Geometry: final body of the model. Coordinates: model frame, mm. Face numbers are marked on the shaded views. A direction names the side the tool comes from. Give positions to 0.01 mm unless a question says otherwise; leave off trailing zeros. Loops run counter-clockwise (first coordinate to the right, second up) from the corner with the lowest first, then second, coordinate; pieces in that order, holes last.
from build123d import *

# Parameters (mm, degrees)
SKETCH4_W                     = 38.1
SKETCH4_H                     = 38.1
BOSS_EXTRUDE2_DEPTH           = 15.24
BOSS_EXTRUDE2_TAPER           = 45
BOSS_EXTRUDE2_OTHER_WAY_DEPTH = 19.05
SKETCH10_W                    = 50.8
SKETCH10_H                    = 50.8
BOSS_EXTRUDE3_DEPTH           = 12.7
BOSS_EXTRUDE3_TAPER           = -45
BOSS_EXTRUDE3_OTHER_WAY_DEPTH = 2.54
BOSS_EXTRUDE3_OTHER_WAY_TAPER = 45


with BuildPart() as part:
    # Sketch4 → Boss-Extrude2 (new body)
    with BuildSketch(Plane(origin=(0, 0, 0), x_dir=(0, 0, -1), z_dir=(1, 0, 0))):
        Rectangle(SKETCH4_W, SKETCH4_H)
    extrude(amount=BOSS_EXTRUDE2_DEPTH, taper=BOSS_EXTRUDE2_TAPER)

    # Sketch4 → Boss-Extrude2 other way (add)
    with BuildSketch(Plane(origin=(0, 0, 0), x_dir=(0, 0, -1), z_dir=(1, 0, 0))):
        Rectangle(SKETCH4_W, SKETCH4_H)
    extrude(amount=-BOSS_EXTRUDE2_OTHER_WAY_DEPTH)

    # Sketch10 → Boss-Extrude3 (add)
    with BuildSketch(Plane.ZY.offset(19.05)):
        Rectangle(SKETCH10_W, SKETCH10_H)
    extrude(amount=BOSS_EXTRUDE3_DEPTH, taper=BOSS_EXTRUDE3_TAPER)

    # Sketch10 → Boss-Extrude3 other way (add)
    with BuildSketch(Plane.ZY.offset(19.05)):
        Rectangle(SKETCH10_W, SKETCH10_H)
    extrude(amount=-BOSS_EXTRUDE3_OTHER_WAY_DEPTH, taper=BOSS_EXTRUDE3_OTHER_WAY_TAPER)


solid = part.part
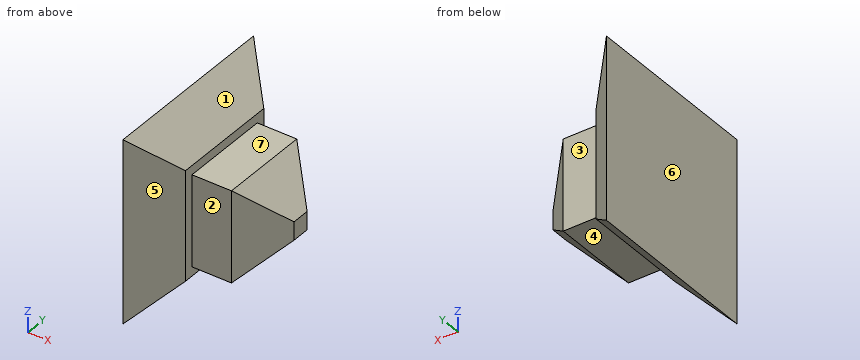
Item 1: Ray query, probe 1 along Y at (x, z) = (-11, 16.5); probe 2 along X at (y, z) = (14, 20.5). Return the intervals inside material, ascending.
Values follow:
probe 1: y = -19.05 to 19.05
probe 2: x = -31.75 to -16.51
Item 2: Draft query along X for the marked faces 5, 6 and 7. Return one class per face: +X half, -X half, draft (parallel to the pull), parting line (faces both ways), or undercut.
Values follow:
face 5: +X half
face 6: -X half
face 7: draft
Item 3: Section query B-B on x = -24. Return loops of the section in (y, z).
Values follow:
outline: (-30.35, -30.35) - (30.35, -30.35) - (30.35, 30.35) - (-30.35, 30.35) - close
Item 4: Set-up query: the marked faces 1, 2, 3 and 4. Return all of +Z, -Z, +X, -X, +Y, -Y with unobstructed straight access to the full face (end or side cutting, diameter ignored); none if empty.
Values follow:
face 1: +Z, +X, +Y, -Y
face 2: +Z, -Z, +X, -Y
face 3: +Z, -Z, +X, +Y
face 4: -Z, +X, +Y, -Y
Item 5: Pin query (flat end, axial travel): pin 1 (1.5 mm diameter, centred on y = -4, z = -15, fed in from +X); pin 2 (4 mm diameter, centred on y = 25, z = -23, fed in from +X); pin 3 (8 mm diameter, centred on y = 16, z = -5.5, fed in from +X). Return the tip coordinate at first contact, or that it passes through.
Values follow:
pin 1: stops at x = 4.8
pin 2: stops at x = -16.65
pin 3: stops at x = 7.05
Item 6: Section query A-A on y = -28. Return loops of the section in (x, z), plus the area to 3 significant figures.
Values follow:
outline: (-31.75, -38.1) - (-21.65, -28) - (-21.65, 28) - (-31.75, 38.1) - close
area: 668 mm2
